Drawing for the job (mm, zero at the part's lowest x, y, z). Coordinates: 2 decimals unless noted, no trailing zeros. Write each loop counter-clockwise with the first axis right and the second up, starting at its lowest first coordinate (ties: lowest second). Pieces come first, ordered by that corner, then holes. Notation, with made-up numbers: M 87,-11 L 93,-11 A8 ccw 93,-7 Z; hole C 23.25,-22 d8. An arc over 180 degrees is marked long. Use a Markdown table: item, result. Add a question column.
Q1. Pin check, flat tips, straight feed: pin 1 Ø4 at (x, z) = (193.5, 14) entering from +Y; pin 2 Ø5 at (y, z) = (17.5, 13.5) entering from -X; pin 3 Ø1.5 at (y, z) = (4, 6.5) entering from +X. Stop position of each tip, or through.
Q2. Wall check: L1, parallel to X at y = 11.25, z = 11.75; L2, parallel to X at y = 14.5, z = 15.25; L3, parallel to X at y = 21, z = 21.25. Give the ranges that are in metal, low to high. Write a range as from..to.
Q3. Slice it at C-C on y = 19.5. Write the cut outline in (x, z).
Q4. Slice it at A-A on y = 7.75. Write the cut outline in (x, z), then the cut area to 3 significant figures.
Q5. Slice it at B-B on z = 12.5. Write the cut outline in (x, y).
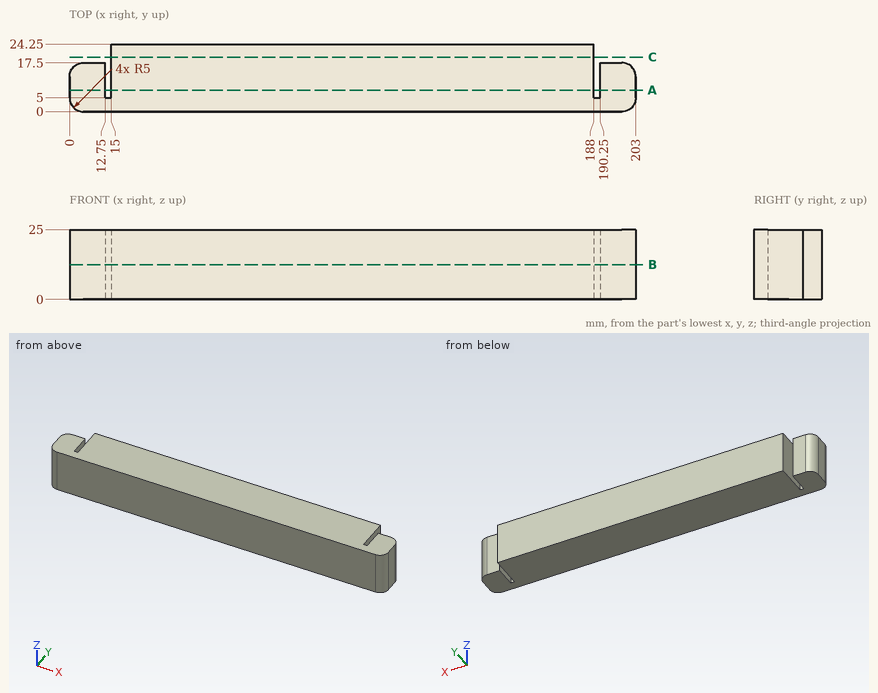
Recorded:
| question | item | result |
|---|---|---|
| 1 | pin 1 | y = 17.5 |
| 1 | pin 2 | x = 0.67 |
| 1 | pin 3 | x = 202.99 |
| 2 | L1 | 0..12.75, 15..188, 190.25..203 |
| 2 | L2 | 0.42..12.75, 15..188, 190.25..202.58 |
| 2 | L3 | 15..188 |
| 3 | outline | M 15,0 L 188,0 L 188,25 L 15,25 Z |
| 4 | outline | M 0,0 L 12.75,0 L 12.75,25 L 0,25 Z; M 15,0 L 188,0 L 188,25 L 15,25 Z; M 190.25,0 L 203,0 L 203,25 L 190.25,25 Z |
| 4 | area | 4,960 mm² |
| 5 | outline | M 0,5 A5 ccw 5,0 L 198,0 A5 ccw 203,5 L 203,12.5 A5 ccw 198,17.5 L 190.25,17.5 L 190.25,5 L 188,5 L 188,24.25 L 15,24.25 L 15,5 L 12.75,5 L 12.75,17.5 L 5,17.5 A5 ccw 0,12.5 Z |
